```python
from build123d import *

# Parameters (mm, degrees)
SKETCH1_R           = 5
BOSS_EXTRUDE1_DEPTH = 20
SKETCH2_R           = 3.5
BOSS_EXTRUDE2_DEPTH = 8
BOSS_EXTRUDE3_START = 8
SKETCH3_R           = 3.5
BOSS_EXTRUDE3_DEPTH = 8
BOSS_EXTRUDE4_DEPTH = 5
BOSS_EXTRUDE5_START = 5
BOSS_EXTRUDE5_DEPTH = 5
SKETCH7_R           = 1.5
CUT_EXTRUDE1_DEPTH  = 15
BOSS_EXTRUDE6_REACH = 43.605
SKETCH8_R           = 4
BOSS_EXTRUDE7_REACH = 43.605
SKETCH9_R           = 4


with BuildPart() as part:
    # Sketch1 → Boss-Extrude1 (new body)
    with BuildSketch(Plane.XY):
        Circle(SKETCH1_R)
    extrude(amount=BOSS_EXTRUDE1_DEPTH)

    # Sketch2 → Boss-Extrude2 (add)
    with BuildSketch(Plane.XY.offset(20)):
        Circle(SKETCH2_R)
    extrude(amount=BOSS_EXTRUDE2_DEPTH)

    # Sketch3 → Boss-Extrude3 (add)
    with BuildSketch(Plane(origin=(0, 0, 0), x_dir=(-1, 0, 0), z_dir=(0, 0, -1)).offset(BOSS_EXTRUDE3_START)):
        with Locations(Location((0, 0, 0), (0, 0, 180))):
            Circle(SKETCH3_R)
    extrude(amount=-BOSS_EXTRUDE3_DEPTH)

    # Sketch4 → Boss-Extrude4 (add)
    with BuildSketch(Plane(origin=(0, 0, -8), x_dir=(-1, 0, 0), z_dir=(0, 0, -1))):
        with BuildLine():
            Line((2.326935409, 0.913986654), (-2.326935409, 0.913986654))
            ThreePointArc((-2.326935409, 0.913986654), (-0.465113684, -2.456352837), (2.5, 0))
            ThreePointArc((2.5, 0), (2.456352837, 0.465113684), (2.326935409, 0.913986654))
        make_face()
    extrude(amount=BOSS_EXTRUDE4_DEPTH)

    # Sketch6 → Boss-Extrude5 (add)
    with BuildSketch(Plane.XY.offset(28).offset(BOSS_EXTRUDE5_START)):
        with BuildLine():
            Line((2.32849737, 0.91), (-2.32849737, 0.91))
            ThreePointArc((-2.32849737, 0.91), (-0.46301003, -2.456750234), (2.5, 0))
            ThreePointArc((2.5, 0), (2.456750234, 0.46301003), (2.32849737, 0.91))
        make_face()
    extrude(amount=-BOSS_EXTRUDE5_DEPTH)

    # Sketch7 → Cut-Extrude1 (cut)
    with BuildSketch(Plane.ZY.offset(5)):
        with Locations((15.5, 0)):
            Circle(SKETCH7_R)
    extrude(amount=-CUT_EXTRUDE1_DEPTH, mode=Mode.SUBTRACT)

    # Sketch8 → Boss-Extrude6 (add, up to next)
    with BuildSketch(Plane(origin=(0, 0, -8), x_dir=(-1, 0, 0), z_dir=(0, 0, -1)), mode=Mode.PRIVATE) as boss_extrude6_sk1:
        Circle(SKETCH8_R)
    boss_extrude6_tool1 = extrude(boss_extrude6_sk1.sketch, amount=-BOSS_EXTRUDE6_REACH, mode=Mode.PRIVATE) - part.part
    add(boss_extrude6_tool1.solids().sort_by_distance((0, 0, -8))[0])

    # Sketch9 → Boss-Extrude7 (add, up to next)
    with BuildSketch(Plane.XY.offset(28), mode=Mode.PRIVATE) as boss_extrude7_sk1:
        with Locations(Location((0, 0, 0), (0, 0, 180))):
            Circle(SKETCH9_R)
    boss_extrude7_tool1 = extrude(boss_extrude7_sk1.sketch, amount=-BOSS_EXTRUDE7_REACH, mode=Mode.PRIVATE) - part.part
    add(boss_extrude7_tool1.solids().sort_by_distance((0, 0, 28))[0])


solid = part.part
```
Design review of the part built by this model. Coordinates are the model's own, in mm. A direction names the side the tool comes from. Coordinates: 2 decimals unless noted, no trailing zeros. Loops run counter-clockwise (first coordinate to the right, second up) from the corner with the lowest first, then second, coordinate; pieces in that order, holes last. Notation, with made-up numbers: M -22.5,80.5 L -11.5,80.5 A24 ccw -11.5,103.5 Z; hole C -28.5,62.5 d10. An arc over 180 degrees is marked long. One line per question, with ' | ' between items.
(1) Draft analysis for pull direction Y (two halves, no side actions). For faces 1 (the face through (0, 0.914, -10)), 2 (the face through (0, 0, 14)), 3 (the face through (0.867, 3.905, 24.056)), 4 (the face through (0, 0, 33)), state which applies: released by +Y, released by -Y, zero draft, split by the parting line, or undercut.
Filled in:
face 1: released by +Y | face 2: undercut | face 3: split by the parting line | face 4: zero draft
(2) We need section B-B (y = 0.5). Give the boundary of the cut face in (x, z), and give its area (3 significant figures).
Filled in:
outline: M -4.97,0 L -3.97,0 L -3.97,-8 L -2.45,-8 L -2.45,-13 L 2.45,-13 L 2.45,-8 L 3.97,-8 L 3.97,0 L 4.97,0 L 4.97,14.09 L -4.97,14.09 Z; M -4.97,16.91 L 4.97,16.91 L 4.97,20 L 3.97,20 L 3.97,28 L 2.45,28 L 2.45,33 L -2.45,33 L -2.45,28 L -3.97,28 L -3.97,20 L -4.97,20 Z | area: 347 mm^2
(3) We need section D-D (z = -5). Give the boundary of the cut face in (x, y), and give its area (3 significant figures).
Filled in:
outline: C 0,0 d8 | area: 50.3 mm^2
(4) Wall thickness on probe 1 along Z at (x, y) = (2, 0); probe 2 along Z at (x, y) = (-2.25, -3.5); probe 3 along Y at (x, z) = (2, 15.5): over which ranges is each line inside the solid? List them lowest first.
Filled in:
probe 1: z = -13 to 14, 17 to 33 | probe 2: z = 0 to 20 | probe 3: y = -4.58 to -1.5, 1.5 to 4.58
(5) We need section C-C (z = 15.5). Give the boundary of the cut face in (x, y).
Filled in:
outline: M -4.77,-1.5 A5 ccw 4.77,-1.5 Z; M -4.77,1.5 L 4.77,1.5 A5 ccw Z
(6) For pin 1 Ø1.5 at (x, z) = (2, 20) entering from +Y; pin 2 Ø5 at (y, z) = (-2, 18.5) entering from +X; pin 3 Ø5 at (x, z) = (-0.5, -11.5) entering from +Y; pin 4 Ø1.5 at (x, z) = (-1.5, 2.5) entering from -Y, all flat-tipped, find the tip position at first contact; note any pin that passes through.
Filled in:
pin 1: stops at y = 4.84 | pin 2: stops at x = 5 | pin 3: stops at y = 0.91 | pin 4: stops at y = -4.94
(7) Machinability: for faces 5 (the face through (0, 0.91, 31)), 6 (the face through (0.867, -3.905, -4.056)), 7 (the face through (0, 2, 28)), which of the approach directions +Z, -Z, +X, -X, +Y, -Y give a long, thin tool a straight path to every point of the face, cutting with its end or side? Answer none if there is none.
Filled in:
face 5: +Z, +X, -X, +Y | face 6: -Z | face 7: +Z
(8) We need section A-A (x = 0). Give the boundary of the cut face in (y, z), and give its area (3 significant figures).
Filled in:
outline: M -5,0 L -4,0 L -4,-8 L -2.5,-8 L -2.5,-13 L 0.91,-13 L 0.91,-8 L 4,-8 L 4,0 L 5,0 L 5,20 L 4,20 L 4,28 L 0.91,28 L 0.91,33 L -2.5,33 L -2.5,28 L -4,28 L -4,20 L -5,20 Z; hole C 0,15.5 d3 | area: 355 mm^2
